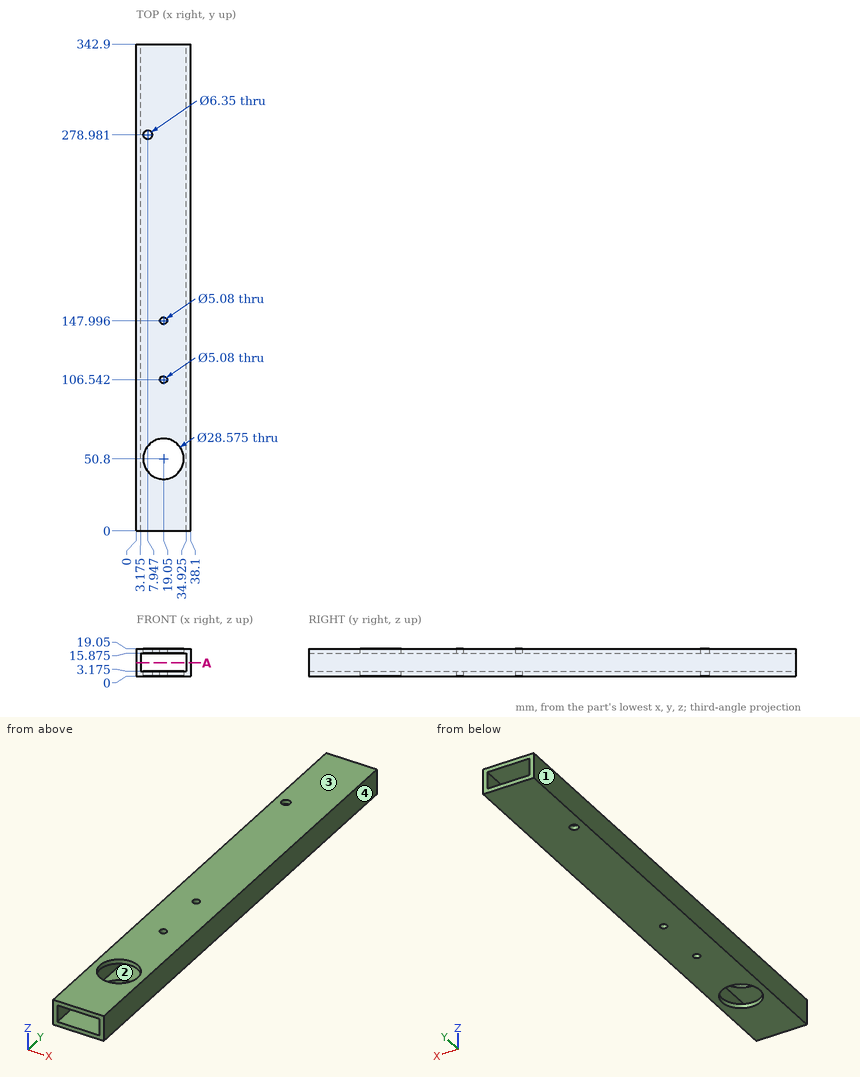
Job drawing, mm, ordinate dimensions from the low corner. One solid piece. Coordinates: 2 decimals unless noted, no trailing zeros. Write each loop counter-clockwise with the first axis right and the second up, starting at its lowest first coordinate (ties: lowest second). Pieces come first, ordered by that corner, then holes. Notation, with made-up numbers: M -13.5,61 L -7.5,61 A7 ccw -7.5,74 Z; hole C 53,-34.75 d3. An arc over 180 degrees is marked long. Answer as a JSON object with one key per item and string values. Group by question number.
1) Wall check: line 1 (Y direction, x = 19.05, z = 0.8); line 2 (X direction, y = 236.5, z = 10) (1 decimal); line 3 (Y direction, x = 27.5, z = 18). Give the ranges that are in metal, low to high. Write a range as from..to.
2) Saw through at A-A (z = 9.25). Write the cut outline in (x, y) (1 decimal).
3) Mould opens along X. For the marked faces 1, 2, 3 and 4 say: +X half, -X half, draft (parallel to the pull), parting line (faces both ways), or undercut.
Values follow:
{
 "1": {"line 1": "y = 0..36.51, 65.09..104, 109.08..145.46, 150.54..342.9", "line 2": "x = 0..3.2, 34.9..38.1", "line 3": "y = 0..39.28, 62.32..342.9"},
 "2": {"outline": "M 0,0 L 3.2,0 L 3.2,342.9 L 0,342.9 Z; M 34.9,0 L 38.1,0 L 38.1,342.9 L 34.9,342.9 Z"},
 "3": {"face 1": "-X half", "face 2": "undercut", "face 3": "draft", "face 4": "+X half"}
}
